Print and shaded views of the part. All mm, measured from the part's lowest x, y and z. A direction names the side the tool comes from. Coordinates: 2 decimals unless noted, no trailing zeros. Loops run counter-clockwise (first coordinate to the right, second up) from the corner with the lowest first, then second, coordinate; pieces in that order, holes last. Notation, with made-up numbers: M 38,66 L 62,66 A4 cw 62,72 Z; hole C 52.5,-29.5 d1. An arc over 180 degrees is marked long. Use a Markdown table: item, result. Add a question column.
1) Band-saw the part on D-D (z = 6). List the corners of the cut face in (x, y).
2) Tool access for the marked faces 1 and 2: list every direction of +Z, -Z, +X, -X, +Y, -Y with a clear straight run to the whole face (end or side of a thin tool).
3) Pin check, flat tips, straight feed: pin 1 Ø8 at (x, z) = (14.5, 40.5) entering from +Y; pin 2 Ø6.5 at (x, z) = (45, 5) entering from +Y. Stop position of each tip, or through.
4) Band-saw the part on B-B (y = 20). List the corners of the cut face in (x, z), plus the area to 3 significant figures.
5) Band-saw the part on A-A (x = 25). List the corners of the cut face in (y, z), plus the area to 3 significant figures.
6) Wall check: probe 1 along Z at (x, y) = (5, 0.6); probe 2 along Y at (x, z) = (36.5, 26.5); probe 3 along Z at (x, y) = (44, 43). Give the ranges that are in metal, low to high. Write a range as from..to.
7) Band-saw the part on C-C (z = 32). List the corners of the cut face in (x, y), plus the area to 3 significant figures.
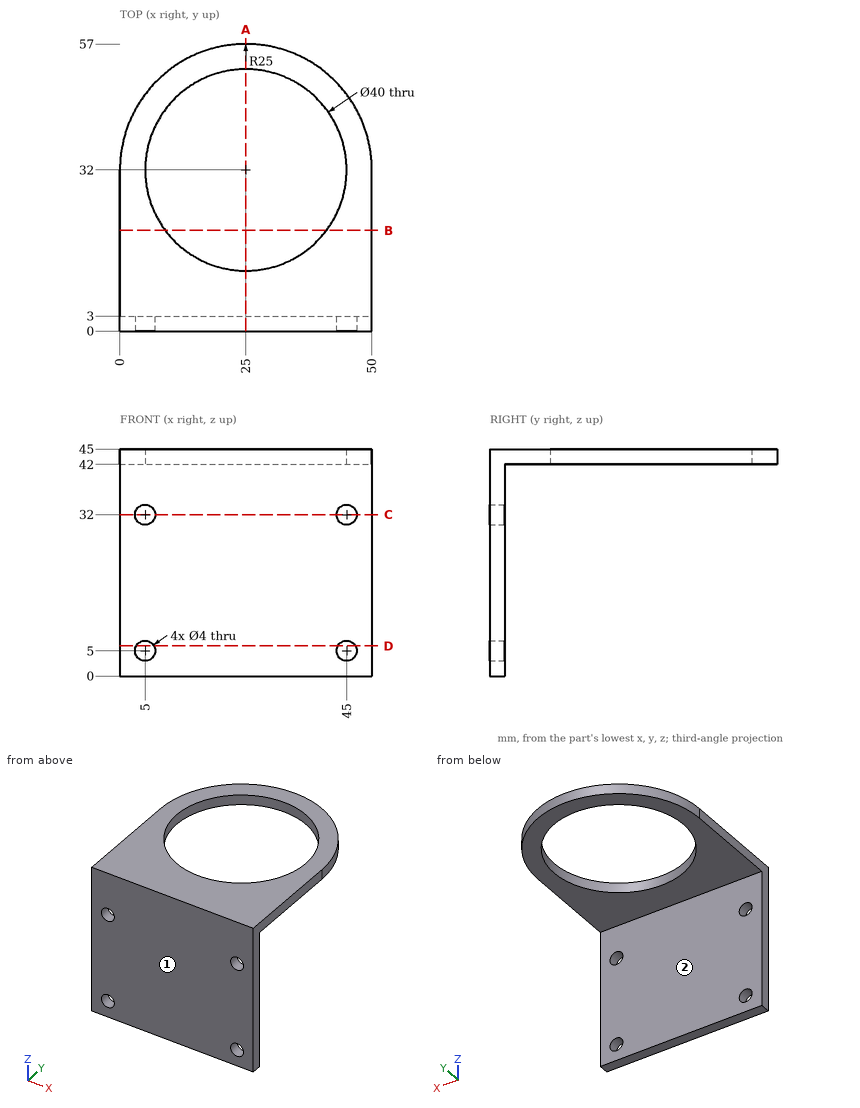
Entries:
| question | item | result |
|---|---|---|
| 1 | outline | M 0,0 L 3.27,0 L 3.27,3 L 0,3 Z; M 6.73,0 L 43.27,0 L 43.27,3 L 6.73,3 Z; M 46.73,0 L 50,0 L 50,3 L 46.73,3 Z |
| 2 | face 1 | +Z, -Z, +X, -X, -Y |
| 2 | face 2 | -Z, +X, -X, +Y |
| 3 | pin 1 | y = 56.06 |
| 3 | pin 2 | y = 3 |
| 4 | outline | M 0,42 L 9,42 L 9,45 L 0,45 Z; M 41,42 L 50,42 L 50,45 L 41,45 Z |
| 4 | area | 54.0 mm2 |
| 5 | outline | M 0,0 L 3,0 L 3,42 L 12,42 L 12,45 L 0,45 Z; M 52,42 L 57,42 L 57,45 L 52,45 Z |
| 5 | area | 177 mm2 |
| 6 | probe 1 | 0..3, 7..30, 34..45 |
| 6 | probe 2 | 0..3 |
| 6 | probe 3 | 42..45 |
| 7 | outline | M 0,0 L 3,0 L 3,3 L 0,3 Z; M 7,0 L 43,0 L 43,3 L 7,3 Z; M 47,0 L 50,0 L 50,3 L 47,3 Z |
| 7 | area | 126 mm2 |
